```python
from build123d import *

# Parameters (mm, degrees)
F0_W     = 23.5
F0_H     = 23.5
F1_DEPTH = 11.75
F2_W     = 22
F2_H     = 22
F3_DEPTH = 50
F4_W     = 22
F4_H     = 22
F5_DEPTH = 50
F6_W     = 22
F6_H     = 22
F7_DEPTH = 50
F8_W     = 22
F8_H     = 22
F9_DEPTH = 50


with BuildPart() as f1:
    # F0 (on Front) → F1 (new body, symmetric)
    with BuildSketch(Plane.XZ):
        Rectangle(F0_W, F0_H)
    extrude(amount=F1_DEPTH, both=True)

    # F2 (on face) → F3 (join)
    with BuildSketch(Plane(origin=(-11.75, 0, 0), x_dir=(0, -1, 0), z_dir=(-1, 0, 0))):
        Rectangle(F2_W, F2_H)
    extrude(amount=F3_DEPTH)

    # F4 (on face) → F5 (join)
    with BuildSketch(Plane.XY.offset(11.75)):
        Rectangle(F4_W, F4_H)
    extrude(amount=F5_DEPTH)

    # F6 (on face) → F7 (join)
    with BuildSketch(Plane.XZ.offset(11.75)):
        Rectangle(F6_W, F6_H)
    extrude(amount=F7_DEPTH)

    # F8 (on face) → F9 (join)
    with BuildSketch(Plane.YZ.offset(11.75)):
        Rectangle(F8_W, F8_H)
    extrude(amount=F9_DEPTH)


solid = f1.part
```
Geometry: final body of the model. Coordinates: model frame, mm. A direction names the side the tool comes from. Coordinates: 2 decimals unless noted, no trailing zeros. Order: outer loops, then holes, each group sorted by start corner. A loop starts at its lowest first (then second) coordinate and runs counter-clockwise, first axis right, second up. Notation, with made-up numbers: (63, 38.5) -> (68, 38.5) arc R22 ccw to (68, 51.5) -> close; hole circle Ø4 at (12, 65.5). An arc over 180 degrees is marked (long way). Answer in a Markdown table with one row per item.
Item 1: Ray query, L1, parallel to X at y = -48.5, z = 9. Return the intervals inside material, ascending.
Return value:
| item | result |
|---|---|
| L1 | x = -11 to 11 |
Item 2: Section C-C on y = 3.5. Output: boundary loops of the cut face in (x, z), plus the area to 3 significant figures.
Return value:
| item | result |
|---|---|
| outline | (-61.75, -11) -> (-11.75, -11) -> (-11.75, -11.75) -> (11.75, -11.75) -> (11.75, -11) -> (61.75, -11) -> (61.75, 11) -> (11.75, 11) -> (11.75, 11.75) -> (11, 11.75) -> (11, 61.75) -> (-11, 61.75) -> (-11, 11.75) -> (-11.75, 11.75) -> (-11.75, 11) -> (-61.75, 11) -> close |
| area | 3,850 mm² |
Item 3: Access query for faces 1 (the flat face through (36, 0, 11)), 2 (the flat face through (0, -36, 11)), 3 (the flat face through (-36, 0, -11)). Directions: +Z, -Z, +X, -X, +Y, -Y. A direction counts if a zero-diameter tool reaches every point of the face in a straight line with its end or side. Return the directions, or none.
Return value:
| item | result |
|---|---|
| face 1 | +Z, +X, +Y, -Y |
| face 2 | +Z, +X, -X, -Y |
| face 3 | -Z, -X, +Y, -Y |
Item 4: Section D-D on z = 38. Output: boundary loops of the cut face in (x, y), plus the area to 3 significant figures.
Return value:
| item | result |
|---|---|
| outline | (-11, -11) -> (11, -11) -> (11, 11) -> (-11, 11) -> close |
| area | 484 mm² |
Item 5: Contact query for flat-ended pins moving along their axis: P1, Ø6.5, axis at x = 3, y = -37, coming from the +Z side; P2, Ø11, axis at y = -47, z = -3, coming from the -X side; P3, Ø17.5, axis at y = 3.5, z = 37.5, coming from the +X side. Output: stop coordinate, or through.
Return value:
| item | result |
|---|---|
| P1 | stops at z = 11 |
| P2 | stops at x = -11 |
| P3 | stops at x = 11 |
Item 6: Section B-B on x = 3. Output: boundary loops of the cut face in (y, z), plus the area to 3 significant figures.
Return value:
| item | result |
|---|---|
| outline | (-61.75, -11) -> (-11.75, -11) -> (-11.75, -11.75) -> (11.75, -11.75) -> (11.75, 11.75) -> (11, 11.75) -> (11, 61.75) -> (-11, 61.75) -> (-11, 11.75) -> (-11.75, 11.75) -> (-11.75, 11) -> (-61.75, 11) -> close |
| area | 2,750 mm² |
Item 7: Section A-A on z = 1.5. Output: boundary loops of the cut face in (x, y).
Return value:
| item | result |
|---|---|
| outline | (-61.75, -11) -> (-11.75, -11) -> (-11.75, -11.75) -> (-11, -11.75) -> (-11, -61.75) -> (11, -61.75) -> (11, -11.75) -> (11.75, -11.75) -> (11.75, -11) -> (61.75, -11) -> (61.75, 11) -> (11.75, 11) -> (11.75, 11.75) -> (-11.75, 11.75) -> (-11.75, 11) -> (-61.75, 11) -> close |
